Design review of the part built by this model. Coordinates are the model's own, in mm. A direction names the side the tool comes from. Give positions to 0.01 mm unless a question says otherwise; leave off trailing zeros. Loops run counter-clockwise (first coordinate to the right, second up) from the corner with the lowest first, then second, coordinate; pieces in that order, holes last. Notation, with made-up numbers: (57, 5) -> (105, 5) arc R29 cw to (105, 41) -> close; hole circle Ø11 at (30.5, -25.75). An arc over 180 degrees is marked (long way). Answer in a Markdown table with one row per item. Add a question column.
(1) Consider section B-B on y = 3. Write out the cut boundary in (x, z).
(2) Draft analysis for pull direction X (two halves, no side actions). For faces 4 (the cylindrical face through (-3.2, 3.6, 0)), 5 (the flat face through (-6, 2, 0)), 6 (the flat face through (0, 3, 8)), state which applies: +X half, -X half, draft (parallel to the pull), parting line (faces both ways), or undercut.
(3) For faces 1 (the flat face through (6, 3, 0)), 2 (the cylindrical face through (4.8, 3.6, 0)), 3 (the flat face through (-2.5, 1, 0)), list the 3-axis set-ups (+Z, -Z, +X, -X, +Y, -Y) from which the entire face can be reached by the end or side of a thin tool; tool diameter is ignored.
(4) For line 1 (X direction, y = 0.4, z = 2.5); line 2 (Z direction, x = -4, y = 3.2); line 3 (X direction, y = 4.7, z = -0.5), list the stretches that pass through material, from the lowest coordinate up.
(5) For pin 1 (1.5 mm diameter, centred on x = 0, z = -2.5, fed in from -Y); pin 2 (2 mm diameter, centred on x = 4, z = 0, fed in from +Y), all flat-tipped, find the tip position at first contact; note any pin that passes through.
(6) Consider section C-C on z = 3.5. Write out the cut boundary in (x, y).
(7) Consider section A-A on y = 0.8. Write out the cut boundary in (x, z).
(8) Consider section D-D on x = -1.25. Write out the cut boundary in (y, z), then the cut area to 3 significant figures.
from build123d import *

# Parameters (mm, degrees)
EXTRUDE_1_DEPTH        = 8
HOLE_WIZARD_M2_1_D     = 1.6
HOLE_WIZARD_M2_1_DEPTH = 2.7
HOLE_WIZARD_M2_1_TIP   = 0.480688495


with BuildPart() as part:
    # 草图1 → 凸台-拉伸1 (new, symmetric)
    with BuildSketch(Plane.XY):
        Polygon((-6, 5), (6, 5), (6, 0), (2.5, 0), (2.5, 2.7), (-2.5, 2.7), (-2.5, 0), (-6, 0), align=None)
    extrude(amount=EXTRUDE_1_DEPTH, both=True)

    # M2 螺纹孔1
    with Locations(Plane(origin=(0, 5, 0), x_dir=(1, 0, 0), z_dir=(0, 1, 0))):
        with Locations((-4, 0), (4, 0)):
            Hole(HOLE_WIZARD_M2_1_D / 2, depth=HOLE_WIZARD_M2_1_DEPTH)
            with Locations((0, 0, -(HOLE_WIZARD_M2_1_DEPTH + HOLE_WIZARD_M2_1_TIP / 2))):  # 118° drill point
                Cone(0, HOLE_WIZARD_M2_1_D / 2, HOLE_WIZARD_M2_1_TIP, mode=Mode.SUBTRACT)


solid = part.part
Values follow:
| question | item | result |
|---|---|---|
| 1 | outline | (-6, -8) -> (6, -8) -> (6, 8) -> (-6, 8) -> close; hole circle Ø1.6 at (-4, 0); hole circle Ø1.6 at (4, 0) |
| 2 | face 4 | undercut |
| 2 | face 5 | -X half |
| 2 | face 6 | draft |
| 3 | face 1 | +Z, -Z, +X, +Y, -Y |
| 3 | face 2 | +Y |
| 3 | face 3 | +Z, -Z, -Y |
| 4 | line 1 | -6 to -2.5, 2.5 to 6 |
| 4 | line 2 | -8 to -0.8, 0.8 to 8 |
| 4 | line 3 | -6 to -4.62, -3.38 to 3.38, 4.62 to 6 |
| 5 | pin 1 | y = 2.7 |
| 5 | pin 2 | y = 5 |
| 6 | outline | (-6, 0) -> (-2.5, 0) -> (-2.5, 2.7) -> (2.5, 2.7) -> (2.5, 0) -> (6, 0) -> (6, 5) -> (-6, 5) -> close |
| 7 | outline | (-6, -8) -> (-2.5, -8) -> (-2.5, 8) -> (-6, 8) -> close; (2.5, -8) -> (6, -8) -> (6, 8) -> (2.5, 8) -> close |
| 8 | outline | (2.7, -8) -> (5, -8) -> (5, 8) -> (2.7, 8) -> close |
| 8 | area | 36.8 mm2 |
